Autodesk Fusion 360 part; units mm, degrees
sketch "Sketch1" plane through (0, 0, 0) normal (0, 1, 0) x (1, 0, 0)
  circle A0 centre (0, 0) radius 7.91
  circle A1 centre (0, 0) radius 3.5
  dimension "d1" = 15.82
  dimension "d2" = 7
extrude "Extrude1" add sketch "Sketch1" along normal blind 3
sketch "Sketch2" plane through (0, 3, 0) normal (0, 1, 0) x (-1, 0, 0)
  circle A0 centre (0, 0) radius 3.5
  circle A1 centre (0, 0) radius 7.91
  circle A2 centre (0, 0) radius 9.6
  dimension "d5" = 19.2
extrude "Extrude2" add sketch "Sketch2" along normal blind 6.932 contours A1 | A2
sketch "Sketch3" plane through (0, 9.932, 0) normal (0, 1, 0) x (-1, 0, 0)
  circle A0 centre (0, 0) radius 3.5
  circle A1 centre (0, 0) radius 9.6
  circle A2 centre (0, 0) radius 5.4
  dimension "d8" = 10.8
extrude "Extrude3" cut sketch "Sketch3" against normal blind 3 contours A2
sketch "Sketch4" plane through (0, 9.932, 0) normal (0, 1, 0) x (-1, 0, 0)
  circle A0 centre (0, 0) radius 5.4
  circle A1 centre (0, 0) radius 9.6
  circle A2 centre (0, 0) radius 8
extrude "Extrude4" cut sketch "Sketch4" against normal blind 5.5 contours A1
extrude "Extrude5" cut 1 faces at (-4.7335, 6.932, -0.4422) along direction (0, -1, 0) blind 2
extrude "Extrude6" cut 1 faces at (-7.0834, 9.932, -0.6657) along direction (0, -1, 0) blind 1
Design review of the part built by this model. Coordinates are the model's own, in mm. A direction names the side the tool comes from. Give positions to 0.01 mm unless a question says otherwise; leave off trailing zeros. Write each loop counter-clockwise with the first axis right and the second up, starting at its lowest first coordinate (ties: lowest second). Pieces come first, ordered by that corner, then holes. Notation, with made-up numbers: (28.5, 22.5) -> (83.5, 22.5) arc R11 cw to (83.5, 29.5) -> close; hole circle Ø7 at (39.25, 7). An arc over 180 degrees is marked (long way). Answer in a Markdown table with one row per item.
(1) Consider section A-A (z = 3). State the section outline as (x, y) points.
Results:
| item | result |
|---|---|
| outline | (-9.12, 3) -> (-7.32, 3) -> (-7.32, 0) -> (-1.8, 0) -> (-1.8, 4.93) -> (-4.49, 4.93) -> (-4.49, 8.93) -> (-7.42, 8.93) -> (-7.42, 4.43) -> (-9.12, 4.43) -> close; (1.8, 0) -> (7.32, 0) -> (7.32, 3) -> (9.12, 3) -> (9.12, 4.43) -> (7.42, 4.43) -> (7.42, 8.93) -> (4.49, 8.93) -> (4.49, 4.93) -> (1.8, 4.93) -> close |
(2) Mouldability with a two-part tool opening along X and no side actions: class faces 1 (the flat face through (-5.22, 8.932, 1.89)), 2 (the flat face through (0, 4.932, -4)), 3 (the cylindrical face through (1.17, 6.96, -5.27)), 4 (the cylindrical face through (-1.715, 1.479, -7.722)) as +X half, -X half, draft (parallel to the pull), parting line (faces both ways), or undercut.
Results:
| item | result |
|---|---|
| face 1 | draft |
| face 2 | undercut |
| face 3 | undercut |
| face 4 | parting line |
(3) Consider section D-D (z = 5). State the section outline as (x, y) points (3 decimals), then the cut area to 3 significant figures.
Results:
| item | result |
|---|---|
| outline | (-8.195, 3) -> (-6.129, 3) -> (-6.129, 0) -> (6.129, 0) -> (6.129, 3) -> (8.195, 3) -> (8.195, 4.432) -> (6.245, 4.432) -> (6.245, 8.932) -> (2.04, 8.932) -> (2.04, 4.932) -> (-2.04, 4.932) -> (-2.04, 8.932) -> (-6.245, 8.932) -> (-6.245, 4.432) -> (-8.195, 4.432) -> close |
| area | 100 mm2 |
(4) Consider section C-C (y = 0.75). State the section outline as (x, z) points.
Results:
| item | result |
|---|---|
| outline | circle Ø15.82 at (0, 0); hole circle Ø7 at (0, 0) |
(5) To check wall thickness, follow probe 1 along Z at (x, y) = (0, 7.2); probe 2 along Z at (x, y) = (0, 2.2); probe 3 along X at (y, z) = (6.25, -1.25). State the ranges of each line that lie inside material, in increasing order.
Results:
| item | result |
|---|---|
| probe 1 | -8 to -5.4, 5.4 to 8 |
| probe 2 | -7.91 to -3.5, 3.5 to 7.91 |
| probe 3 | -7.9 to -5.25, 5.25 to 7.9 |
(6) Clearance check with flat-ended pins moving along their axes: pin 1 (2 mm diameter, centred on y = 1, z = -0.5, fed in from +X); pin 2 (5.5 mm diameter, centred on x = 0.5, z = 2, fed in from +Y); pin 3 (1 mm diameter, centred on x = -6, y = 4.5, fed in from +Z). State where each tip first meets the part, or that it passes through.
Results:
| item | result |
|---|---|
| pin 1 | x = 7.91 |
| pin 2 | y = 4.93 |
| pin 3 | z = 7.87 |
(7) For faces 5 (the cylindrical face through (1.73, 6.71, -7.81)), 6 (the flat face through (3.4, 0, 1.6)), 7 (the flat face through (-1, 3, 8)), list the 3-axis set-ups (+Z, -Z, +X, -X, +Y, -Y) from which the entire face can be reached by the end or side of a thin tool; tool diameter is ignored.
Results:
| item | result |
|---|---|
| face 5 | +Y |
| face 6 | +Z, -Z, +X, -X, -Y |
| face 7 | -Y |
